Build history of the part. All positions in model axes, mm. Face numbers are marked on the shaded views. A direction names the side the tool comes from. Coordinates: 2 decimals unless noted, no trailing zeros. Order: outer loops, then holes, each group sorted by start corner. A loop starts at its lowest first (then second) coordinate and runs counter-clockwise, first axis right, second up. Notation, with made-up numbers: M 67.5,13.5 L 115.5,13.5 A9 ccw 115.5,18.5 Z; hole C -23.75,-39.75 d8. An arc over 180 degrees is marked long. Write item = value, one per line. Start each with the question number.
Q1. 3-axis set-ups, long thin cutter, end or side, ignore diameter. For the marked faces 4 and 5: which of +Z, -Z, +X, -X, +Y, -Y reach the whole face in a straight line?
Q2. Band-saw the part on C-C on y = 28. Write the cut outline in (x, z).
Q3. Pin check, flat tips, straight feed: P1, Ø0.8, axis at x = 12, y = 29.5, coming from the -Z side; P2, Ø6, axis at x = 20.5, y = 23.5, coming from the +Z side; P3, Ø1.8, axis at x = 1.5, y = 19, coming from the +Z side. Stop position of each tip, or through.
Q4. Drill centre lines: probe 1 along Y at (x, z) = (6.5, 2.7); probe 2 along X at (y, z) = (15.75, 2.8); probe 3 along Y at (x, z) = (15, 1.4). Where is each one in solid material? Low to high.
Q5. Band-saw the part on A-A on x = 6.5. Write the cut outline in (y, z).
Q6. Band-saw the part on D-D on x = 17.5. Write the cut outline in (y, z).
Q7. Pull direction Y, two halves, no side cores. Call the marked faces 1, 2 and 3: released by +Y, released by -Y, zero draft, split by the parting line, or undercut.
Q8. Band-saw the part on B-B on z = -1.6. Write the cut outline in (x, y), plus the area to 3 significant figures.
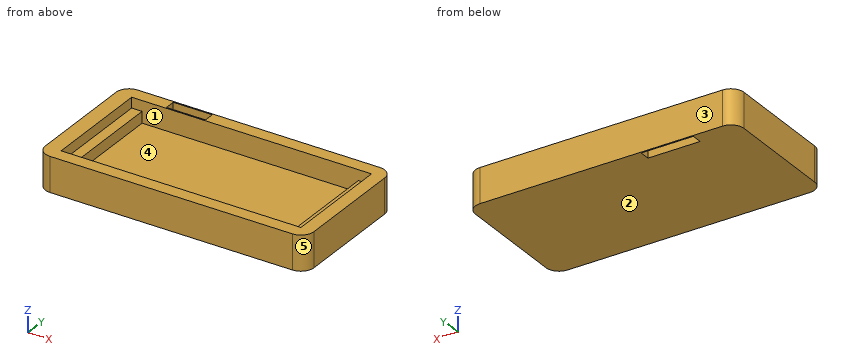
```python
from build123d import *

# Parameters (mm, degrees)
CROQUIS1_W              = 37.22
CROQUIS1_H              = 16.7
SALIENTE_EXTRUIR1_DEPTH = 3.35
VACIADO1_T              = 2
REDONDEO1_R             = 2
CROQUIS2_W              = 2
CROQUIS2_H              = 16.7
SALIENTE_EXTRUIR2_DEPTH = 1.75
CROQUIS6_W              = 0.4
CROQUIS6_H              = 16.7
SALIENTE_EXTRUIR5_DEPTH = 1.6
CROQUIS7_W              = 6
CROQUIS7_H              = 1.6
CORTAR_EXTRUIR1_DEPTH   = 3
CROQUIS10_W             = 8
CROQUIS10_H             = 1.6
CORTAR_EXTRUIR2_DEPTH   = 3


with BuildPart() as part:
    # Croquis1 → Saliente-Extruir1 (new body)
    with BuildSketch(Plane.XY):
        with Locations((18.552250715, 20.301071835)):
            Rectangle(CROQUIS1_W, CROQUIS1_H)
    extrude(amount=SALIENTE_EXTRUIR1_DEPTH)

    # Vaciado1
    vaciado1_openings = [part.faces().sort_by_distance(p)[0] for p in [
        (18.552250715, 20.301071835, 3.35),
    ]]
    offset(amount=VACIADO1_T, openings=vaciado1_openings, kind=Kind.INTERSECTION)

    # Redondeo1
    # the kernel refuses this fillet: 2 mm, written as the material it takes off along each edge
    with BuildSketch(Plane(origin=(-2.057749285, 30.651071835, -7), x_dir=(1, 0, 0), z_dir=(0, 0, 1)), Plane(origin=(39.162250715, 30.651071835, 8.35), x_dir=(-1, 0, 0), z_dir=(0, 0, -1)), Plane(origin=(39.162250715, 9.951071835, 8.35), x_dir=(0, 1, 0), z_dir=(0, 0, -1)), Plane(origin=(-2.057749285, 9.951071835, 8.35), x_dir=(1, 0, 0), z_dir=(0, 0, -1))) as redondeo1_piece_1:
        with BuildLine():
            CenterArc((REDONDEO1_R, -REDONDEO1_R), REDONDEO1_R, 90, 90)
            Line((0, -REDONDEO1_R), (0, 0))
            Line((0, 0), (REDONDEO1_R, 0))
        make_face()
    extrude(amount=15.35, mode=Mode.SUBTRACT)

    # Croquis2 → Saliente-Extruir2 (add)
    with BuildSketch(Plane.XY):
        with Locations((0.942250715, 20.301071835)):
            Rectangle(CROQUIS2_W, CROQUIS2_H)
        with Locations((36.162250715, 20.301071835)):
            Rectangle(CROQUIS2_W, CROQUIS2_H)
    extrude(amount=SALIENTE_EXTRUIR2_DEPTH)

    # Croquis6 → Saliente-Extruir5 (add)
    with BuildSketch(Plane.XY.offset(1.75)):
        with Locations((0.142250715, 20.301071835)):
            Rectangle(CROQUIS6_W, CROQUIS6_H)
    extrude(amount=SALIENTE_EXTRUIR5_DEPTH)

    # Croquis7 → Cortar-Extruir1 (cut)
    with BuildSketch(Plane.XY.offset(3.35)):
        with Locations((8.552250715, 29.651071835)):
            Rectangle(CROQUIS7_W, CROQUIS7_H)
    extrude(amount=-CORTAR_EXTRUIR1_DEPTH, mode=Mode.SUBTRACT)

    # Croquis10 → Cortar-Extruir2 (cut)
    with BuildSketch(Plane.XY.offset(0.35)):
        with Locations((8.552250715, 29.651071835)):
            Rectangle(CROQUIS10_W, CROQUIS10_H)
    extrude(amount=-CORTAR_EXTRUIR2_DEPTH, mode=Mode.SUBTRACT)


solid = part.part
```
Recorded:
q1.face_4 = +Z
q1.face_5 = +Z, -Z, +X, -Y
q2.outline = M -2.06,-2 L 39.16,-2 L 39.16,3.35 L 37.16,3.35 L 37.16,1.75 L 35.16,1.75 L 35.16,0 L 1.94,0 L 1.94,1.75 L 0.34,1.75 L 0.34,3.35 L -2.06,3.35 Z
q3.P1 = 0.35
q3.P2 = 0
q3.P3 = 1.75
q4.probe_1 = 9.95 to 11.95, 28.65 to 28.85, 30.45 to 30.65
q4.probe_2 = -2.06 to 0.34, 37.16 to 39.16
q4.probe_3 = 9.95 to 11.95, 28.65 to 30.65
q5.outline = M 9.95,-2 L 28.85,-2 L 28.85,3.35 L 28.65,3.35 L 28.65,0 L 11.95,0 L 11.95,3.35 L 9.95,3.35 Z; M 30.45,-2 L 30.65,-2 L 30.65,3.35 L 30.45,3.35 Z
q6.outline = M 9.95,-2 L 30.65,-2 L 30.65,3.35 L 28.65,3.35 L 28.65,0 L 11.95,0 L 11.95,3.35 L 9.95,3.35 Z
q7.face_1 = undercut
q7.face_2 = zero draft
q7.face_3 = released by +Y
q8.outline = M -2.06,11.95 A2 ccw -0.06,9.95 L 37.16,9.95 A2 ccw 39.16,11.95 L 39.16,28.65 A2 ccw 37.16,30.65 L -0.06,30.65 A2 ccw -2.06,28.65 Z; hole M 4.55,28.85 L 12.55,28.85 L 12.55,30.45 L 4.55,30.45 Z
q8.area = 837 mm2
